from build123d import *

# Parameters (mm, degrees)
SKETCH_1_W          = 48.184
SKETCH_1_H          = 28.88
SKETCH_1_W_2        = 1
SKETCH_1_H_2        = 23.68
EXTRUDE_1_DEPTH     = 2
EXTRUDE_2_DEPTH     = 11.4
SKETCH_1_7_W        = 53.184
SKETCH_1_7_H        = 33.88
SKETCH_1_7_W_2      = 50.184
SKETCH_1_7_H_2      = 30.88
EXTRUDE_3_DEPTH     = 11
SKETCH_2_W          = 3.8
SKETCH_2_H          = 21
CUT_EXTRUDE_1_DEPTH = 62.941490586
SKETCH_3_W          = 5
SKETCH_3_H          = 10
SKETCH_3_W_2        = 9
SKETCH_3_H_2        = 13
CUT_EXTRUDE_2_DEPTH = 62.109575813
FILLET_1_R          = 0.8
CHAMFER_1_SIZE      = 0.4
SKETCH_4_R          = 2
CUT_EXTRUDE_3_DEPTH = 1.2
SKETCH_4_3_W        = 2
SKETCH_4_3_H        = 8
EXTRUDE_4_DEPTH     = 8


with BuildPart() as part:
    # Эскиз1 → Бобышка-Вытянуть1 (new body)
    with BuildSketch(Plane.XY):
        with Locations((24.892, 15.24)):
            Rectangle(SKETCH_1_W, SKETCH_1_H)
        with Locations((49.484, 17.84)):
            Rectangle(SKETCH_1_W_2, SKETCH_1_H_2)
    extrude(amount=-EXTRUDE_1_DEPTH)

    # Эскиз1<6> → Бобышка-Вытянуть2 (add)
    with BuildSketch(Plane.XY):
        Polygon((0.8, 29.68), (48.984, 29.68), (49.984, 29.68), (49.984, 30.68), (-0.2, 30.68), (-0.2, -0.2), (49.984, -0.2), (49.984, 6), (48.984, 6), (48.984, 0.8), (0.8, 0.8), align=None)
    extrude(amount=-EXTRUDE_2_DEPTH)

    # Эскиз1<7> → Бобышка-Вытянуть3 (add)
    with BuildSketch(Plane.XY):
        with Locations((24.892, 15.24)):
            Rectangle(SKETCH_1_7_W, SKETCH_1_7_H)
        with Locations((24.892, 15.24)):
            Rectangle(SKETCH_1_7_W_2, SKETCH_1_7_H_2, mode=Mode.SUBTRACT)
    extrude(amount=-EXTRUDE_3_DEPTH)

    # Эскиз2 → Вырез-Вытянуть1 (cut, through all)
    with BuildSketch(Plane.ZY.offset(-49.984)):
        with Locations((-9.1, 18.37)):
            Rectangle(SKETCH_2_W, SKETCH_2_H)
    extrude(amount=-CUT_EXTRUDE_1_DEPTH, mode=Mode.SUBTRACT)

    # Эскиз3 → Вырез-Вытянуть2 (cut, through all)
    with BuildSketch(Plane(origin=(0.8, 0, 0), x_dir=(0, 0, -1), z_dir=(1, 0, 0))):
        with Locations((8.9, 24.5)):
            Rectangle(SKETCH_3_W, SKETCH_3_H)
        with Locations((6.9, 8.25)):
            Rectangle(SKETCH_3_W_2, SKETCH_3_H_2)
    extrude(amount=-CUT_EXTRUDE_2_DEPTH, mode=Mode.SUBTRACT)

    # Скругление1
    fillet_1_edges = [part.edges().sort_by_distance(p)[0] for p in [
        (-0.45, 29.5, -6.4),
        (-0.45, 19.5, -6.4),
        (-0.45, 14.75, -2.4),
        (-0.45, 1.75, -2.4),
        (50.734, 28.87, -7.2),
        (50.734, 7.87, -7.2),
    ]]
    fillet(fillet_1_edges, radius=FILLET_1_R)

    # Фаска1
    chamfer_1_edges = [part.edges().sort_by_distance(p)[0] for p in [
        (-0.2, 0.775, -11.4),
        (24.892, -0.2, -11.4),
        (49.984, 2.9, -11.4),
        (49.984, 30.18, -11.4),
        (24.892, 30.68, -11.4),
        (-0.2, 30.09, -11.4),
        (-0.2, 17.125, -11.4),
    ]]
    chamfer(chamfer_1_edges, length=CHAMFER_1_SIZE - 0.0001)  # a hair under: the kernel refuses the full size

    # Эскиз4 → Вырез-Вытянуть3 (cut)
    with BuildSketch(Plane(origin=(0, 0, -2), x_dir=(-1, 0, 0), z_dir=(0, 0, -1))):
        with Locations((-40.9, 27.6)):
            Circle(SKETCH_4_R)
        with Locations((-27.6, 27.6)):
            Circle(SKETCH_4_R)
        with Locations((-11.8, 2.8)):
            Circle(SKETCH_4_R)
    extrude(amount=-CUT_EXTRUDE_3_DEPTH, mode=Mode.SUBTRACT)

    # Эскиз4<3> → Бобышка-Вытянуть4 (add)
    with BuildSketch(Plane(origin=(0, 0, -2), x_dir=(-1, 0, 0), z_dir=(0, 0, -1))):
        with Locations((-34.3, 25.68)):
            Rectangle(SKETCH_4_3_W, SKETCH_4_3_H)
    extrude(amount=EXTRUDE_4_DEPTH)


solid = part.part
Verification items for the finished model (mm, model axes). A direction names the side the tool comes from. Round coordinates to 2 decimals unless told otherwise and drop trailing zeros. Loops run counter-clockwise (first coordinate to the right, second up) from the corner with the lowest first, then second, coordinate; pieces in that order, holes last. Notation, with made-up numbers: (-12.5, 85.5) - (43.5, 85.5) arc R30 cw to (43.5, 121.5) - close; hole circle Ø7 at (-23.5, 36.25). An arc over 180 degrees is marked (long way). Use a Markdown table: item, result. Add a question column.
1. Access from +Z, -Z, +X, -X, +Y, -Y to the whole of each face (thin tool, end or side, straight path). Record for faces 3 (the face through (0, 1.75, -7)), 4 (the face through (-1, 17, -11)), 5 (the face through (41.16, 29.583, -1.408)).
2. Section check A-A, the plane z = -5.25. Record the boundary of the cut face in (x, y).
3. Thickness scan on probe 1 along Y at (x, z) = (40.9, -1.15); probe 2 along Y at (x, z) = (16, -7.5); probe 3 along X at (y, z) = (24.5, -7). Record the ranges inside material, lowest first. Write a range as [from, to].
4. Gauge pin test, flat ends, axial feed: pin 1 (4 mm diameter, centred on x = 45.5, y = 12.5, fed in from -Z); pin 2 (3 mm diameter, centred on x = 40.9, y = 27.6, fed in from -Z); pin 3 (1.6 mm diameter, centred on x = 51, y = 23, fed in from -Z). Record the tip position at first contact, or that the pin passes through.
5. Release check for a two-part mould opening along Y. For faces 1 (the face through (24.8, 0.5, -11.4)), 2 (the face through (33.3, 26, -6)) record: released by +Y, released by -Y, zero draft, split by the parting line, or undercut.
Checks:
| question | item | result |
|---|---|---|
| 1 | face 3 | -Z, -X |
| 1 | face 4 | -Z, -X, +Y, -Y |
| 1 | face 5 | -Z |
| 2 | outline | (-1.7, -1.7) - (51.48, -1.7) - (51.48, 32.18) - (-1.7, 32.18) - (-1.7, 14.75) - (0.8, 14.75) - (0.8, 29.68) - (33.3, 29.68) - (33.3, 21.68) - (35.3, 21.68) - (35.3, 29.68) - (49.98, 29.68) - (49.98, 6) - (48.98, 6) - (48.98, 0.8) - (0.8, 0.8) - (0.8, 1.75) - (-1.7, 1.75) - close |
| 3 | probe 1 | y = [-1.7, 25.6], [29.6, 32.18] |
| 3 | probe 2 | y = [-1.7, 0.8], [29.68, 32.18] |
| 3 | probe 3 | x = [33.3, 35.3], [49.98, 51.48] |
| 4 | pin 1 | stops at z = -2 |
| 4 | pin 2 | stops at z = -0.8 |
| 4 | pin 3 | stops at z = -7.2 |
| 5 | face 1 | zero draft |
| 5 | face 2 | undercut |
